Part model, mm, in its own coordinate system. Face numbers are marked on the shaded views. A direction names the side the tool comes from. Round coordinates to 2 decimals unless told otherwise and drop trailing zeros. Write each loop counter-clockwise with the first axis right and the second up, starting at its lowest first coordinate (ties: lowest second). Pieces come first, ordered by that corner, then holes. Notation, with made-up numbers: (19, 10.25) -> (61, 10.25) arc R19 cw to (61, 32.25) -> close; hole circle Ø9 at (84, -17). An arc over 180 degrees is marked (long way). Return JSON: item names as keys, results as strings. Group by question number.
(1) Drop a flat-ended pin along its axis: pin 1 Ø1.5 at (y, z) = (-1, -3.5) entering from -X. Give the stop position or say it passes through.
(2) Tool access for the marked faces 1 and 2: list every direction of +Z, -Z, +X, -X, +Y, -Y with a clear straight run to the whole face (end or side of a thin tool).
(3) Drill centre lines: L1, parallel to Y at x = 24.5, z = 0; L2, parallel to Y at x = 28.5, z = -4; L3, parallel to Z at x = 12, y = -0.25. Where is each one in solid material? Low to high. Write a range as from..to.
(4) Saw through at A-A (x = 32). List the corners of the cut face in (y, z).
(5) Saw through at B-B (x = 8). List the corners of the cut face in (y, z).
from build123d import *

# Parameters (mm, degrees)
FILLET1_R = 0.5


with BuildPart() as part:
    # Sketch1 → Revolve1 (revolve)
    with BuildSketch(Plane.XY, mode=Mode.PRIVATE) as revolve1_sk:
        Polygon((0, 0), (0, 4.5), (0.5, 5), (34.5, 5), (35, 4.5), (35, 0), align=None)
    revolve(revolve1_sk.sketch.rotate(Axis((35, 0, 0), (-1, 0, 0)), 270), axis=Axis((35, 0, 0), (-1, 0, 0)))

    # Sketch2 → Revolve2 (revolve)
    with BuildSketch(Plane.XY, mode=Mode.PRIVATE) as revolve2_sk:
        Polygon((-8, 0), (-8, 2.3865), (-7.3865, 3), (0, 3), (0, 0), align=None)
    revolve(revolve2_sk.sketch.rotate(Axis((0, 0, 0), (-1, 0, 0)), 270), axis=Axis((0, 0, 0), (-1, 0, 0)))

    # Sketch3 → Cut-Revolve1 (revolve, cut)
    with BuildSketch(Plane.XY, mode=Mode.PRIVATE) as cut_revolve1_sk:
        Polygon((20.5, 0), (21.209852156, 1.2295), (34.7295, 1.2295), (35, 1.5), (35, 0), align=None)
    revolve(cut_revolve1_sk.sketch.rotate(Axis((35, 0, 0), (-1, 0, 0)), 270), axis=Axis((35, 0, 0), (-1, 0, 0)), mode=Mode.SUBTRACT)

    # Sketch5 → Cut-Revolve2 (revolve, cut)
    with BuildSketch(Plane(origin=(0, 0, 0), x_dir=(1, 0, 0), z_dir=(0, 1, 0)), mode=Mode.PRIVATE) as cut_revolve2_sk:
        Polygon((0, 3), (1.678199262, 5), (0, 5), align=None)
    revolve(cut_revolve2_sk.sketch.rotate(Axis((0, 0, 0), (1, 0, 0)), 180), axis=Axis((0, 0, 0), (1, 0, 0)), mode=Mode.SUBTRACT)

    # Fillet1
    fillet1_edges = [part.edges().sort_by_distance(p)[0] for p in [
        (1.678199262, 0, -5),
    ]]
    fillet(fillet1_edges, radius=FILLET1_R)


solid = part.part
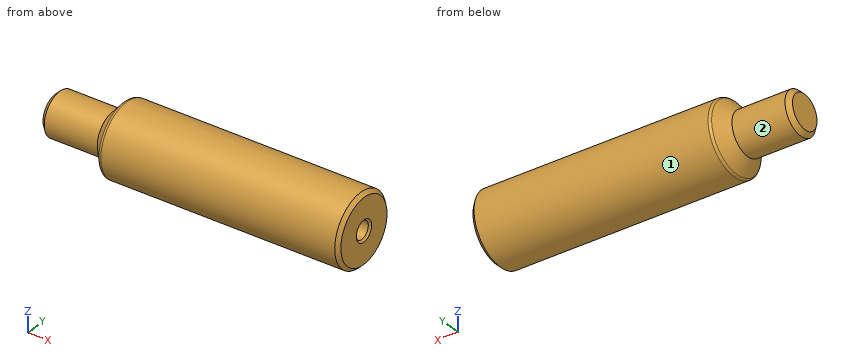
Computed values:
{
 "1": {"pin 1": "x = -7.5"},
 "2": {"face 1": "+X, -X", "face 2": "-X"},
 "3": {"L1": "-5..-1.23, 1.23..5", "L2": "-3..3", "L3": "-4.99..4.99"},
 "4": {"outline": "circle Ø10 at (0, 0); hole circle Ø2.46 at (0, 0)"},
 "5": {"outline": "circle Ø10 at (0, 0)"}
}
